Source: CAD feature listing. Evaluate the final solid. Frame: model axes, mm. Face numbers are marked on the shaded views. A direction names the side the tool comes from. Give positions to 0.01 mm unless a question says otherwise; leave off trailing zeros. Order: outer loops, then holes, each group sorted by start corner. A loop starts at its lowest first (then second) coordinate and runs counter-clockwise, first axis right, second up.
1) Section A-A, the plane y = -33. Return loops of the section in (x, z).
2) Access query for the marked faces 1, 2 and 3. Directions: +Z, -Z, +X, -X, +Y, -Y. A direction counts if a zero-diameter tool reaches every point of the face in a straight line with its end or side. Return the directions, or none.
3) Section B-B, the plane x = -40. Return loops of the section in (y, z).
4) Section D-D, the plane x = -68.5. Return loops of the section in (y, z), plus the area to 3 significant figures.
5) Section C-C, the plane z = 9. Return loops of the section in (x, y).
6) Material intervals for line 1 (Y direction, x = -40, z = 24.75); line 2 (Z direction, x = -75, y = -23.5); line 3 (Y direction, x = -51, z = 14), sorted ascending.
7) Draft query along Y for the marked faces 4, 5 and 6. Return one class per face: released by +Y, released by -Y, zero draft, split by the parting line, or undercut.
8) First-contact query: P1, Ø9.5, axis at x = -45.5, y = -41.5, coming from the -Z side; P2, Ø2, axis at y = -40.5, z = 10, coming from the +X side; P3, Ø4.5, axis at x = -92, y = -76, coming from the +Z side. Flat tips, straight axial feed; report the tip coordinate or a pass-through.
```python
from build123d import *

# Parameters (mm, degrees)
F0_W      = 100
F0_H      = 45
F1_DEPTH  = 80
F2_R      = 7.5
F3_DEPTH  = 30
F5_DEPTH  = 20
F6_W      = 20
F6_H      = 15
F7_DEPTH  = 10
F10_DEPTH = 80.001
F11_DEPTH = 25


with BuildPart() as f1:
    # F0 (on Front) → F1 (new body)
    with BuildSketch(Plane.XZ):
        with Locations((-50, 22.5)):
            Rectangle(F0_W, F0_H)
    extrude(amount=F1_DEPTH)

    # F2 (on face) → F3 (cut)
    with BuildSketch(Plane.XY.offset(45)):
        with Locations((-40, -15)):
            Circle(F2_R)
    extrude(amount=-F3_DEPTH, mode=Mode.SUBTRACT)

    # F4 (on face) → F5 (cut)
    with BuildSketch(Plane.XY.offset(45)):
        with BuildLine():
            Line((-100, -80), (-30, -80))
            ThreePointArc((-30, -80), (-50.5025253169, -30.5025253169), (-100, -10))
            Line((-100, -10), (-100, -80))
        make_face()
    extrude(amount=-F5_DEPTH, mode=Mode.SUBTRACT)

    # F6 (on face) → F7 (join)
    with BuildSketch(Plane.XY.offset(25)):
        with Locations((-90, -72.5)):
            Rectangle(F6_W, F6_H)
    extrude(amount=F7_DEPTH)

    # F9 (on face) → F10 (cut, through all)
    with BuildSketch(Plane.XZ.offset(80)):
        with BuildLine():
            ThreePointArc((-16.3809735262, 45), (-4.2226032243, 23.944395449), (0, 0))
            Line((0, 0), (0, 45))
            Line((0, 45), (-16.3809735262, 45))
        make_face()
    extrude(amount=-F10_DEPTH, mode=Mode.SUBTRACT)

    # F8 (on face) → F11 (cut)
    with BuildSketch(Plane(origin=(0, 0, 0), x_dir=(1, 0, 0), z_dir=(0, 0, -1))):
        with BuildLine():
            Line((-34, 50), (-65, 50))
            Line((-65, 50), (-65, 19))
            ThreePointArc((-65, 19), (-43.0796897832, 28.0796897832), (-34, 50))
        make_face()
    extrude(amount=-F11_DEPTH, mode=Mode.SUBTRACT)


solid = f1.part
```
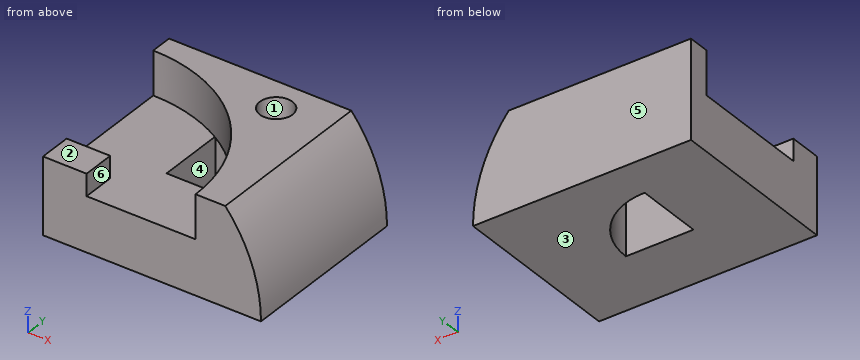
From the geometry:
1. outline: (-100, 0) - (-65, 0) - (-65, 25) - (-100, 25) - close; (-48.13, 25) - (-39.08, 25) - (-39.08, 0) - (0, 0) arc R70 ccw to (-16.38, 45) - (-48.13, 45) - close
2. face 1: +Z
2. face 2: +Z, -X, -Y
2. face 3: -Z, +X, -X, +Y, -Y
3. outline: (-80, 0) - (-50, 0) - (-50, 25) - (-80, 25) - close; (-43.94, 25) - (-31.67, 25) - (-31.67, 0) - (0, 0) - (0, 45) - (-7.5, 45) - (-7.5, 15) - (-22.5, 15) - (-22.5, 45) - (-43.94, 45) - close
4. outline: (-80, 0) - (0, 0) - (0, 45) - (-17.49, 45) - (-17.49, 25) - (-80, 25) - close
4. area: 2,350 mm2
5. outline: (-100, -80) - (-0.58, -80) - (-0.58, 0) - (-100, 0) - close; hole (-65, -50) - (-34, -50) arc R31 ccw to (-65, -19) - close
6. line 1: y = -80 to -50, -31.67 to -22.5, -7.5 to 0
6. line 2: z = 0 to 25
6. line 3: y = -80 to -50, -22.34 to 0
7. face 4: undercut
7. face 5: released by +Y
7. face 6: zero draft
8. P1: stops at z = 25
8. P2: stops at x = -0.58
8. P3: stops at z = 35
